Model file for the job. Use its own axes, mm. Face numbers are marked on the shaded views. A direction names the side the tool comes from. Coordinates: 2 decimals unless noted, no trailing zeros. Order: outer loops, then holes, each group sorted by start corner. A loop starts at its lowest first (then second) coordinate and runs counter-clockwise, first axis right, second up. Notation, with made-up numbers: (33, -9.75) -> (58, -9.75) arc R9 cw to (58, 5.25) -> close; hole circle Ø3 at (43.25, 77). An arc over 180 degrees is marked (long way). Write item = value, one per line. Start each with the question number.
Q1. Mould opens along X. For the marked faces 3, 4 and 5 say: +X half, -X half, draft (parallel to the pull), parting line (faces both ways), or undercut.
Q2. Flat gauge pin, fed straight in: pin 1 (3 mm diameter, centred on x = 30.5, z = 34, fed in from -Y). Where does the tip first touch, or does it go through?
Q3. Cut at B-B, the plane z = 12. List the corners of the cut face in (x, y), plus the area to 3 significant figures.
Q4. Cut at A-A, the plane x = 29.5. List the corners of the cut face in (y, z).
Q5. Wall check: line 1 (Z direction, x = 32, y = -39); line 2 (Y direction, x = 34, z = 37.5). Give the ranges that are in metal, low to high. Write a range as from..to.
Q6. 3-axis set-ups, long thin cutter, end or side, ignore diameter. For the marked faces 1 and 2: which of +Z, -Z, +X, -X, +Y, -Y reach the whole face in a straight line?
from build123d import *

# Parameters (mm, degrees)
ESQUISSE1_W             = 42
ESQUISSE1_H             = 42
BOSS_EXTRU_1_DEPTH      = 42
ESQUISSE2_W             = 10.5
ESQUISSE2_H             = 10.5
ENL_V_MAT_EXTRU_1_DEPTH = 4.5
CONG_1_R                = 0.5


with BuildPart() as part:
    # Esquisse1 → Boss.-Extru.1 (new body)
    with BuildSketch(Plane.XY):
        with Locations((21, -21)):
            Rectangle(ESQUISSE1_W, ESQUISSE1_H)
    extrude(amount=BOSS_EXTRU_1_DEPTH)

    # Esquisse2 → Enlèv. mat.-Extru.1 (cut)
    with BuildSketch(Plane.XZ.offset(42)):
        with Locations((33, 33)):
            Rectangle(ESQUISSE2_W, ESQUISSE2_H)
        with Locations((33, 9)):
            Rectangle(ESQUISSE2_W, ESQUISSE2_H)
    enl_v_mat_extru_1 = extrude(amount=-ENL_V_MAT_EXTRU_1_DEPTH, mode=Mode.SUBTRACT)

    # Congé1
    cong_1_edges = [part.edges().sort_by_distance(p)[0] for p in [
        (42, -21, 42),
        (21, 0, 42),
        (0, -21, 42),
        (21, 0, 0),
        (42, -21, 0),
        (21, -42, 0),
        (0, -21, 0),
        (21, -42, 42),
        (0, 0, 21),
        (42, 0, 21),
        (42, -42, 21),
        (0, -42, 21),
    ]]
    fillet(cong_1_edges, radius=CONG_1_R)

    # Symétrie1: Enlèv. mat.-Extru.1 across plane
    add(enl_v_mat_extru_1.mirror(Plane(origin=(21, 0, 0), x_dir=(0, 0, 1), z_dir=(1, 0, 0))), mode=Mode.SUBTRACT)


solid = part.part
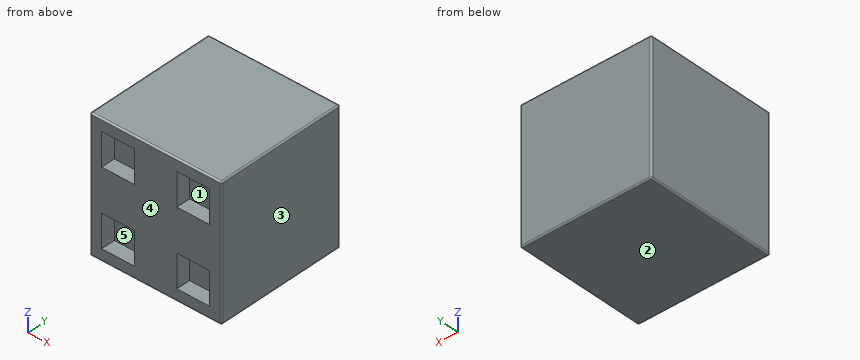
Here are the results:
q1.face_3 = +X half
q1.face_4 = draft
q1.face_5 = undercut
q2.pin_1 = -37.5
q3.outline = (0, -41.5) arc R0.5 ccw to (0.5, -42) -> (3.75, -42) -> (3.75, -37.5) -> (14.25, -37.5) -> (14.25, -42) -> (27.75, -42) -> (27.75, -37.5) -> (38.25, -37.5) -> (38.25, -42) -> (41.5, -42) arc R0.5 ccw to (42, -41.5) -> (42, -0.5) arc R0.5 ccw to (41.5, 0) -> (0.5, 0) arc R0.5 ccw to (0, -0.5) -> close
q3.area = 1,670 mm²
q4.outline = (-42, 0.5) arc R0.5 ccw to (-41.5, 0) -> (-0.5, 0) arc R0.5 ccw to (0, 0.5) -> (0, 41.5) arc R0.5 ccw to (-0.5, 42) -> (-41.5, 42) arc R0.5 ccw to (-42, 41.5) -> (-42, 38.25) -> (-37.5, 38.25) -> (-37.5, 27.75) -> (-42, 27.75) -> (-42, 14.25) -> (-37.5, 14.25) -> (-37.5, 3.75) -> (-42, 3.75) -> close
q5.line_1 = 0..3.75, 14.25..27.75, 38.25..42
q5.line_2 = -37.5..0
q6.face_1 = -Y
q6.face_2 = -Z, +X, -X, +Y, -Y
